Can you work these out from the model? Positions are in its coordinate system, mm. Face numbers are marked on the shaded views. A direction names the side the tool comes from. Give positions to 0.01 mm unless a question says otherwise; leave off trailing zeros. Order: outer loops, then holes, each group sorted by start corner. A loop starts at its lowest first (then second) coordinate and runs counter-clockwise, first axis right, second up. Notation, with made-up numbers: (73.25, 50.25) - (88.25, 50.25) arc R18 ccw to (88.25, 58.25) - close; hole circle Ø8 at (42, 50). An arc over 180 degrees is marked (long way). One line per question, with ' | ' between items.
Autodesk Inventor part; units mm, degrees
ref_plane "YZ Plane" through (0, 0, 0) normal (1, 0, 0) x (0, 1, 0)
ref_plane "XZ Plane" through (0, 0, 0) normal (0, 1, 0) x (-1, 0, 0)
ref_plane "XY Plane" through (0, 0, 0) normal (0, 0, 1) x (1, 0, 0)
sketch "Sketch1" plane through (0, 0, 0) normal (0, 0, 1) x (1, 0, 0)
  line L0 (0, 0) -> (12.7, 0)
  line L1 (12.7, 0) -> (12.7, 134.874)
  line L2 (12.7, 134.874) -> (0, 134.874)
  line L3 (0, 134.874) -> (0, 0)
  line L4 (0, 0) -> (2.54, 0)
  line L5 (2.54, 0) -> (2.54, -12.7)
  line L6 (2.54, -12.7) -> (0, -12.7)
  line L7 (0, -12.7) -> (0, 0)
  dimension "d0" = 12.7
  dimension "d1" = 134.874
  dimension "d2" = 12.7
  dimension "d3" = 2.54
revolve "Revolution1" add sketch "Sketch1" angle 360 about axis through (0, 134.874, 0) along (0, -1, 0)
sketch "Sketch4" plane through (0, 134.874, 0) normal (0, 1, 0) x (1, 0, 0)
  line L0 (3.175, -12.7) -> (3.175, 12.7)
  line L1 (3.175, 12.7) -> (-3.175, 12.7)
  line L2 (-3.175, 12.7) -> (-3.175, -12.7)
  line L3 (-3.175, -12.7) -> (3.175, -12.7)
  line L4 (3.175, -12.7) -> (-3.175, 12.7) construction
  line L5 (3.175, 12.7) -> (-3.175, -12.7) construction
  point P0 (0, 0)
  dimension "d24" = 6.35
  dimension "d25" = 25.4
sketch "Sketch5" plane through (0, 134.874, 0) normal (0, 1, 0) x (1, 0, 0)
  line L0 (-3.2918, -12.7) -> (-12.7, -12.7)
  line L1 (-12.7, -12.7) -> (-12.7, 12.7)
  line L2 (-12.7, 12.7) -> (-3.2918, 12.7)
  line L3 (-3.2918, 12.7) -> (-3.2918, -12.7)
  line L4 (3.4651, -12.7) -> (12.7, -12.7)
  line L5 (12.7, -12.7) -> (12.7, 12.7)
  line L6 (12.7, 12.7) -> (3.4651, 12.7)
  line L7 (3.4651, 12.7) -> (3.4651, -12.7)
  point P0 (0, 0)
extrude "Extrusion2" cut sketch "Sketch5" against normal blind 38.1
sketch "Sketch6" plane through (3.4651, 134.874, 12.2181) normal (1, 0, 0) x (0, 0, -1)
  line L0 (-0.4819, -134.874) -> (24.9181, -134.874)
  line L1 (24.4841, 0) -> (-0.0478, 0)
  point P0 (12.2181, -134.874)
  point P1 (12.2181, -12.7)
  dimension "d39" = 12.7
hole "Hole2" at (3.4651, 122.174, 0) direction (-1, 0, 0) diameter 5.08 end through all
chamfer "Chamfer3" distance 1.27 angle 45 12 edges at (10.1316, 96.774, -7.6578) (10.1316, 96.774, 7.6578) (3.4651, 115.824, -12.2181) (3.4651, 115.824, 12.2181) (3.4651, 134.874, 0) (0.0899, 134.874, -12.6997) (0.0899, 134.874, 12.6997) (-3.2918, 134.874, 0) (-3.2918, 115.824, -12.266) (-3.2918, 115.824, 12.266) (-12.7, 96.774, 0) (-2.54, -12.7, 0)
sketch "Sketch7" plane through (0, -12.7, 0) normal (0, -1, 0) x (1, 0, 0)
  circle A0 centre (0, 0) radius 2.54
  circle A1 centre (0, 0) radius 2.54
  point P0 (0, 0)
extrude "Extrusion3" cut sketch "Sketch7" against normal blind 12.7
sketch "Sketch8" plane through (0, 0, 0) normal (0, -1, 0) x (1, 0, 0)
  point P0 (0, 0)
  point P1 (0, 0)
hole "Hole3" at (0, 0, 0) direction (0, 1, 0) diameter 4.9784 depth 19.05 tip angle 118
properties part number "2016.07.14 magnetic height guide"
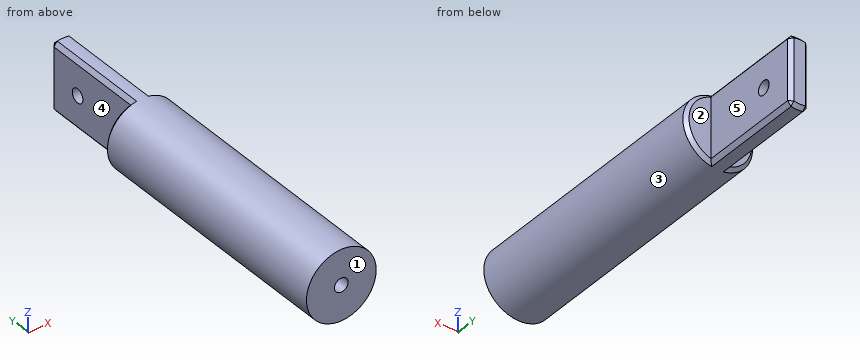
(1) If we mould it in two halves opening along Y, with no side actions, what happens to the marked faces 1, 2 and 3? For each: released by +Y, released by -Y, zero draft, split by the parting line, or undercut.
Answer below:
face 1: released by -Y | face 2: released by +Y | face 3: zero draft
(2) Will these pins go through, and if not, where does the flat tip stop? pin 1 (6.5 mm diameter, centred on x = 8.5, z = 4.5, fed in from +Y); pin 2 (2 mm diameter, centred on y = 114, z = 10, fed in from +X); pin 3 (1 mm diameter, centred on x = -4.5, y = 29.5, fed in from +Z).
Answer below:
pin 1: y = 96.77 | pin 2: x = 3.47 | pin 3: z = 12.05
(3) Imagine slicing it at A-A (y = 79.5). List the corners of the cut face in (x, z) for me.
Answer below:
outline: circle Ø25.4 at (0, 0)
(4) On a 3-axis mill with a long thin cutter (end or side, diameter ignored), from which of +Z, -Z, +X, -X, +Y, -Y can I reach the whole of each face in a straight line? I mean the marked faces 4 and 5. Say none if no direction works.
Answer below:
face 4: +Z, -Z, -X, +Y | face 5: +Z, -Z, +X, +Y
(5) If I drill on line 1 (Z direction, x = 0, y = 7.75), over which ranges is the centre line in solid material (lowest first)?
Answer below:
line 1: -12.7 to -2.49, 2.49 to 12.7
